```python
from build123d import *

# Parameters (mm, degrees)
SKETCH1_W                    = 214
SKETCH1_H                    = 174
BASE_FLANGE1_DEPTH           = 1
EDGE_FLANGE3_STRIP_W         = 5
EDGE_FLANGE3_STRIP_H         = 1
EDGE_FLANGE3_STRIP_CUT_DEPTH = 174
EDGE_FLANGE3_DEPTH           = 174
EDGE_FLANGE4_STRIP_W         = 5
EDGE_FLANGE4_STRIP_H         = 1
EDGE_FLANGE4_STRIP_CUT_DEPTH = 174
EDGE_FLANGE4_DEPTH           = 174
EDGE_FLANGE5_STRIP_W         = 5
EDGE_FLANGE5_STRIP_H         = 1
EDGE_FLANGE5_STRIP_CUT_DEPTH = 41.5
EDGE_FLANGE5_DEPTH           = 41.5
EDGE_FLANGE6_STRIP_W         = 5
EDGE_FLANGE6_STRIP_H         = 1
EDGE_FLANGE6_STRIP_CUT_DEPTH = 41.5
EDGE_FLANGE6_DEPTH           = 41.5
FILLET1_R                    = 4
CUT_EXTRUDE1_REACH           = 161.834
SKETCH24_W                   = 214
SKETCH24_H                   = 2.5
SKETCH26_R                   = 2.5
CUT_EXTRUDE2_DEPTH           = 10
CHAMFER1_SIZE                = 1
CUT_EXTRUDE8_DEPTH           = 219.682418132
CUT_EXTRUDE9_DEPTH           = 254.158053397
FILLET2_R                    = 5


# Sheet-metal steps are written as plain solids
with BuildPart() as part:
    # Sketch1 → Base-Flange1 (new body)
    with BuildSketch(Plane(origin=(0, 0, 0), x_dir=(1, 0, 0), z_dir=(0, 1, 0))):
        Rectangle(SKETCH1_W, SKETCH1_H)
    extrude(amount=-BASE_FLANGE1_DEPTH)

    # Edge-Flange3 strip (across the edge) → Edge-Flange3 strip cut (cut)
    with BuildSketch(Plane(origin=(-107, 0, -87), x_dir=(1, 0, 0), z_dir=(0, 0, 1))):
        with Locations((-1, -0.5)):
            Rectangle(EDGE_FLANGE3_STRIP_W, EDGE_FLANGE3_STRIP_H)
    extrude(amount=EDGE_FLANGE3_STRIP_CUT_DEPTH, mode=Mode.SUBTRACT)

    # Edge-Flange3 section (across the edge) → Edge-Flange3 (add)
    with BuildSketch(Plane(origin=(-107, 0, -87), x_dir=(1, 0, 0), z_dir=(0, 0, 1))):
        with BuildLine():
            Line((0, 0.5), (0, 42))
            Line((0, 42), (1, 42))
            Line((1, 42), (1, 0.5))
            ThreePointArc((1, 0.5), (1.146446609, 0.146446609), (1.5, 0))
            Line((1.5, 0), (1.5, -1))
            ThreePointArc((1.5, -1), (0.439339828, -0.560660172), (0, 0.5))
        make_face()
    extrude(amount=EDGE_FLANGE3_DEPTH)

    # Edge-Flange4 strip (across the edge) → Edge-Flange4 strip cut (cut)
    with BuildSketch(Plane(origin=(107, 0, 87), x_dir=(-1, 0, 0), z_dir=(0, 0, -1))):
        with Locations((-1, -0.5)):
            Rectangle(EDGE_FLANGE4_STRIP_W, EDGE_FLANGE4_STRIP_H)
    extrude(amount=EDGE_FLANGE4_STRIP_CUT_DEPTH, mode=Mode.SUBTRACT)

    # Edge-Flange4 section (across the edge) → Edge-Flange4 (add)
    with BuildSketch(Plane(origin=(107, 0, 87), x_dir=(-1, 0, 0), z_dir=(0, 0, -1))):
        with BuildLine():
            Line((0, 0.5), (0, 42))
            Line((0, 42), (1, 42))
            Line((1, 42), (1, 0.5))
            ThreePointArc((1, 0.5), (1.146446609, 0.146446609), (1.5, 0))
            Line((1.5, 0), (1.5, -1))
            ThreePointArc((1.5, -1), (0.439339828, -0.560660172), (0, 0.5))
        make_face()
    extrude(amount=EDGE_FLANGE4_DEPTH)

    # Edge-Flange5 strip (across the edge) → Edge-Flange5 strip cut (cut)
    with BuildSketch(Plane(origin=(107, 42, 87), x_dir=(0, 0, -1), z_dir=(0, -1, 0))):
        with Locations((-1, -0.5)):
            Rectangle(EDGE_FLANGE5_STRIP_W, EDGE_FLANGE5_STRIP_H)
    extrude(amount=EDGE_FLANGE5_STRIP_CUT_DEPTH, mode=Mode.SUBTRACT)

    # Edge-Flange5 section (across the edge) → Edge-Flange5 (add)
    with BuildSketch(Plane(origin=(107, 42, 87), x_dir=(0, 0, -1), z_dir=(0, -1, 0))):
        with BuildLine():
            Line((0, 0.5), (0, 20))
            Line((0, 20), (1, 20))
            Line((1, 20), (1, 0.5))
            ThreePointArc((1, 0.5), (1.146446609, 0.146446609), (1.5, 0))
            Line((1.5, 0), (1.5, -1))
            ThreePointArc((1.5, -1), (0.439339828, -0.560660172), (0, 0.5))
        make_face()
    extrude(amount=EDGE_FLANGE5_DEPTH)

    # Edge-Flange6 strip (across the edge) → Edge-Flange6 strip cut (cut)
    with BuildSketch(Plane(origin=(-107, 0.5, 87), x_dir=(0, 0, -1), z_dir=(0, 1, 0))):
        with Locations((-1, -0.5)):
            Rectangle(EDGE_FLANGE6_STRIP_W, EDGE_FLANGE6_STRIP_H)
    extrude(amount=EDGE_FLANGE6_STRIP_CUT_DEPTH, mode=Mode.SUBTRACT)

    # Edge-Flange6 section (across the edge) → Edge-Flange6 (add)
    with BuildSketch(Plane(origin=(-107, 0.5, 87), x_dir=(0, 0, -1), z_dir=(0, 1, 0))):
        with BuildLine():
            Line((0, 0.5), (0, 20))
            Line((0, 20), (1, 20))
            Line((1, 20), (1, 0.5))
            ThreePointArc((1, 0.5), (1.146446609, 0.146446609), (1.5, 0))
            Line((1.5, 0), (1.5, -1))
            ThreePointArc((1.5, -1), (0.439339828, -0.560660172), (0, 0.5))
        make_face()
    extrude(amount=EDGE_FLANGE6_DEPTH)

    # Fillet1
    fillet1_edges = [part.edges().sort_by_distance(p)[0] for p in [
        (127, 42, 86.5),
        (127, 0.5, 86.5),
        (-127, 0.5, 86.5),
        (-127, 42, 86.5),
    ]]
    fillet(fillet1_edges, radius=FILLET1_R)

    # Cut-Extrude1: up to this face of the body (flat: up to its plane)
    cut_extrude1_end = Plane(part.part.faces().sort_by_distance((114.980552593, 0.5, 86.497536063))[0])
    # Sketch24 → Cut-Extrude1 (cut, up to the picked face)
    with BuildSketch(Plane.XZ.offset(1), mode=Mode.PRIVATE) as cut_extrude1_sk1:
        with Locations((0, 85.75)):
            Rectangle(SKETCH24_W, SKETCH24_H)
    cut_extrude1_tool1 = split(extrude(cut_extrude1_sk1.sketch, amount=-CUT_EXTRUDE1_REACH, mode=Mode.PRIVATE), bisect_by=cut_extrude1_end, keep=Keep.BOTH, mode=Mode.PRIVATE)
    add(cut_extrude1_tool1.solids().sort_by(Axis((0, -1, 85.75), (0, 1, 0)))[0], mode=Mode.SUBTRACT)

    # Sketch26 → Cut-Extrude2 (cut)
    with BuildSketch(Plane.XY.offset(87)):
        with Locations((-118, 37)):
            Circle(SKETCH26_R)
        with Locations((-118, 5.24)):
            Circle(SKETCH26_R)
        with Locations((-118, 21.12)):
            Circle(SKETCH26_R)
        with Locations(Location((118, 5.24, 0), (0, 0, 180))):
            Circle(SKETCH26_R)
        with Locations(Location((118, 21.12, 0), (0, 0, 180))):
            Circle(SKETCH26_R)
        with Locations(Location((118, 37, 0), (0, 0, 180))):
            Circle(SKETCH26_R)
    extrude(amount=-CUT_EXTRUDE2_DEPTH, mode=Mode.SUBTRACT)

    # Chamfer1
    chamfer1_edges = [part.edges().sort_by_distance(p)[0] for p in [
        (-106.5, 42, -87),
        (106.5, 42, -87),
    ]]
    chamfer(chamfer1_edges, length=CHAMFER1_SIZE)

    # Sketch32 → Cut-Extrude8 (cut, through all)
    with BuildSketch(Plane(origin=(0, 0, 86), x_dir=(-1, 0, 0), z_dir=(0, 0, -1))):
        with BuildLine():
            Line((117.5, 39.5), (118.5, 39.5))
            ThreePointArc((118.5, 39.5), (121, 37), (118.5, 34.5))
            Line((118.5, 34.5), (117.5, 34.5))
            ThreePointArc((117.5, 34.5), (115, 37), (117.5, 39.5))
        make_face()
        with BuildLine():
            Line((117.5, 23.62), (118.5, 23.62))
            ThreePointArc((118.5, 23.62), (121, 21.12), (118.5, 18.62))
            Line((118.5, 18.62), (117.5, 18.62))
            ThreePointArc((117.5, 18.62), (115, 21.12), (117.5, 23.62))
        make_face()
        with BuildLine():
            Line((117.5, 7.74), (118.5, 7.74))
            ThreePointArc((118.5, 7.74), (121, 5.24), (118.5, 2.74))
            Line((118.5, 2.74), (117.5, 2.74))
            ThreePointArc((117.5, 2.74), (115, 5.24), (117.5, 7.74))
        make_face()
    cut_extrude8 = extrude(amount=-CUT_EXTRUDE8_DEPTH, mode=Mode.SUBTRACT)

    # Mirror1: Cut-Extrude8 across plane
    add(cut_extrude8.mirror(Plane(origin=(0, 0, 0), x_dir=(0, 0, 1), z_dir=(1, 0, 0))), mode=Mode.SUBTRACT)

    # Sketch41 → Cut-Extrude9 (cut, through all)
    with BuildSketch(Plane.ZY.offset(107)):
        Polygon((-87, 27), (72, 42), (-87, 42), align=None)
    extrude(amount=-CUT_EXTRUDE9_DEPTH, mode=Mode.SUBTRACT)

    # Fillet2
    # the kernel refuses this fillet: 5 mm, written as the material it takes off along each edge
    with BuildSketch(Plane(origin=(105.411683458, 42, 72), x_dir=(0, -0.09392259459562911, -0.9955795027140852), z_dir=(1, 0, 0))) as fillet2_piece_1:
        with BuildLine():
            CenterArc((FILLET2_R * 0.0470653233649, -FILLET2_R), FILLET2_R, 90, 5.38931176)
            Line((-FILLET2_R * 0.0468572712307, -FILLET2_R * 0.00442049728592), (0, 0))
            Line((0, 0), (FILLET2_R * 0.0470653233649, 0))
        make_face()
    extrude(amount=2.176633084, mode=Mode.SUBTRACT)
    with BuildSketch(Plane(origin=(-107.588316542, 42, 72), x_dir=(0, 0, 1), z_dir=(1, 0, 0))) as fillet2_piece_2:
        with BuildLine():
            CenterArc((FILLET2_R * 0.0470653233649, FILLET2_R), FILLET2_R, 264.61068824, 5.38931176)
            Line((-FILLET2_R * 0.0468572712307, FILLET2_R * 0.00442049728592), (0, 0))
            Line((0, 0), (FILLET2_R * 0.0470653233649, 0))
        make_face()
    extrude(amount=2.176633084, mode=Mode.SUBTRACT)
    with BuildSketch(Plane(origin=(94.623743722, 27, -87), x_dir=(0, -1, 0), z_dir=(1, 0, 0))) as fillet2_piece_3:
        with BuildLine():
            CenterArc((FILLET2_R * 0.910100502204, -FILLET2_R), FILLET2_R, 90, 84.61068824)
            Line((-FILLET2_R * 0.0854790005098, -FILLET2_R * 0.906077405404), (0, 0))
            Line((0, 0), (FILLET2_R * 0.910100502204, 0))
        make_face()
    extrude(amount=23.752512555, mode=Mode.SUBTRACT)
    with BuildSketch(Plane(origin=(-118.376256278, 27, -87), x_dir=(0, 0.0939225945956684, 0.9955795027140816), z_dir=(1, 0, 0))) as fillet2_piece_4:
        with BuildLine():
            CenterArc((FILLET2_R * 0.910100502204, FILLET2_R), FILLET2_R, 185.38931176, 84.61068824)
            Line((-FILLET2_R * 0.0854790005098, FILLET2_R * 0.906077405404), (0, 0))
            Line((0, 0), (FILLET2_R * 0.910100502204, 0))
        make_face()
    extrude(amount=23.752512555, mode=Mode.SUBTRACT)


solid = part.part
```
The listing builds one solid part. Answer for the finished solid, in the listing's coordinates (mm). A direction names the side the tool comes from. Round coordinates to 2 decimals unless told otherwise and drop trailing zeros. Order: outer loops, then holes, each group sorted by start corner. A loop starts at its lowest first (then second) coordinate and runs counter-clockwise, first axis right, second up. Notation, with made-up numbers: (-13.75, 18) -> (20.25, 18) arc R29 cw to (20.25, 44) -> close; hole circle Ø7 at (57, 3.5). An arc over 180 degrees is marked (long way). Answer as CSV lines item,"result". Start each with the question number.
(1) The part is cut by section D-D (z = -64). Determine the outline of the cut face in (x, y).
(2) The part is cut by section B-B (z = 40). Determine the outline of the cut face in (x, y).
(3) The part is cut by section A-A (y = 15.5). Determine the outline of the cut face in (x, z).
(4) A tool of negligible diameter and unlimited length cuts with its end or side. For faces 1 (the face through (113, 22, 86)), 2 (the face through (-113, 21, 87)), 3 (the face through (-107, 16, -2)), 4 (the face through (-1, -1, -2)), 5 (the face through (-1, 0, -2)), from which of +Z, -Z, +X, -X, +Y, -Y can it reach the whole face along a straight path? Write none if from no direction.
(5) The part is cut by section C-C (x = -94). Determine the outline of the cut face in (y, z).
(6) Flat-ended cylindrical pins translate along their axes: pin 1 Ø1.2 at (x, z) = (117.5, 85.5) entering from -Y; pin 2 Ø12 at (y, z) = (30.5, -18) entering from -X; pin 3 Ø5 at (y, z) = (20, -66.5) entering from +X. Find the tip coordinate at first contact, or state that the pin passes through.
(7) Find the intervals of material crossed by probe 1 along X at (y, z) = (28, 16); probe 2 along Y at (x, z) = (-71.5, 31.5), in increasing order. Write a range as from..to.
Evaluation:
1,outline,"(-107, 0.5) arc R1.5 ccw to (-105.5, -1) -> (105.5, -1) arc R1.5 ccw to (107, 0.5) -> (107, 29.17) -> (106, 29.17) -> (106, 0.5) arc R0.5 cw to (105.5, 0) -> (-105.5, 0) arc R0.5 cw to (-106, 0.5) -> (-106, 29.17) -> (-107, 29.17) -> close"
2,outline,"(-107, 0.5) arc R1.5 ccw to (-105.5, -1) -> (105.5, -1) arc R1.5 ccw to (107, 0.5) -> (107, 38.98) -> (106, 38.98) -> (106, 0.5) arc R0.5 cw to (105.5, 0) -> (-105.5, 0) arc R0.5 cw to (-106, 0.5) -> (-106, 38.98) -> (-107, 38.98) -> close"
3,outline,"(-127, 86) -> (-107.5, 86) arc R0.5 cw to (-107, 85.5) -> (-107, -87) -> (-106, -87) -> (-106, 85.5) arc R1.5 ccw to (-107.5, 87) -> (-127, 87) -> close; (106, -87) -> (107, -87) -> (107, 85.5) arc R0.5 cw to (107.5, 86) -> (127, 86) -> (127, 87) -> (107.5, 87) arc R1.5 ccw to (106, 85.5) -> close"
4,face 1,"-Z, +X, +Y, -Y"
4,face 2,"+Z, +X, -X, +Y, -Y"
4,face 3,"-Z, -X, +Y, -Y"
4,face 4,"+Z, -Z, +X, -X, -Y"
4,face 5,"+Z, -Z, +Y"
5,outline,"(-1, -87) -> (0, -87) -> (0, 84.5) -> (-1, 84.5) -> close"
6,pin 1,"y = 0.5"
6,pin 2,"x = -107"
6,pin 3,"x = 107"
7,probe 1,"-107..-106, 106..107"
7,probe 2,"-1..0"
